Source: CAD feature listing. Evaluate the final solid. Frame: model axes, mm. A direction names the side the tool comes from. Coordinates: 2 decimals unless noted, no trailing zeros. Loops run counter-clockwise (first coordinate to the right, second up) from the corner with the lowest first, then second, coordinate; pieces in that order, holes last.
Item 1: Section query A-A, the plane x = 9. Return the cut outline in (y, z), then the cut area to 3 significant figures.
Item 2: Line query: probe 1 along Y at (x, z) = (9, 5.3); probe 2 along Z at (x, y) = (2.5, 135.5); probe 3 along Y at (x, z) = (9, 0.85). Output: solid intervals per line, ascending.
Item 3: Section query C-C, the plane y = 10. Return the cut outline in (x, z), then the cut area to 3 significant figures.
Item 4: Section query D-D, the plane x = 22.5. Return the cut outline in (y, z).
Item 5: Pull-direction query (X, two-part tool) for faces 6 (the cylindrical face through (8.874, 18.202, 1.812)), 7 (the cylindrical face through (7.568, 140.906, 4.535)), 8 (the flat face through (9, 125, 2)), 9 (the cylindrical face through (16, 1, 3)); classes: +X half, -X half, draft (parallel to the pull), parting line (faces both ways), or undercut.
Item 6: Pin query (flat end, axial travel): pin 1 Ø3.5 at (y, z) = (16, 3.5) entering from +X; pin 2 Ø4 at (y, z) = (102, 4.5) entering from -X; pin 3 Ø0.8 at (x, y) = (14.5, 135.5) entering from +Z. Return the tip coordinate at first contact, or that it passes through.
Item 7: Section query B-B, the plane y = 130. Return the cut outline in (x, z), then the cut area to 3 significant figures.
Item 8: Reachability of faces 1 (the flat face through (9, 8, 2.5)), 2 (the flat face through (18, 14, 3)), 3 (the flat face through (0, 14, 3)), 4 (the flat face through (9, 86, 7)), 5 (the flat face through (9, 8, 4.5)) from +Z, -Z, +X, -X, +Y, -Y: full face, straight path, thin tool, end or side. Return the list, or none.
```python
from build123d import *

# Parameters (mm, degrees)
ESQUISSE1_R             = 4.5
ESQUISSE1_W             = 18
ESQUISSE1_H             = 20
BOSS_EXTRU_1_DEPTH      = 7
ESQUISSE2_R             = 11
ENL_V_MAT_EXTRU_1_DEPTH = 5
ESQUISSE3_R             = 0.5
BOSS_EXTRU_2_DEPTH      = 3
ESQUISSE4_W             = 18
ESQUISSE4_H             = 20
ENL_V_MAT_EXTRU_2_DEPTH = 2.5
ESQUISSE5_W             = 18
ESQUISSE5_H             = 20
ENL_V_MAT_EXTRU_3_DEPTH = 2.5
CONG_1_R                = 5
CONG_2_R                = 15


with BuildPart() as part:
    # Esquisse1 → Boss.-Extru.1 (new body)
    # profile 1 of 2: a face of its own
    with BuildSketch(Plane.XY):
        Polygon((18, 20), (28, 150), (18, 150), (0, 150), (-10, 150), (0, 20), align=None)
        with Locations((9, 130)):
            Circle(ESQUISSE1_R, mode=Mode.SUBTRACT)
    # profile 2 of 2: a face of its own
    with BuildSketch(Plane.XY):
        with Locations((9, 10)):
            Rectangle(ESQUISSE1_W, ESQUISSE1_H)
    extrude(amount=BOSS_EXTRU_1_DEPTH)

    # Esquisse2 → Enlèv. mat.-Extru.1 (cut)
    with BuildSketch(Plane.XY.offset(7)):
        with Locations((9, 130)):
            Circle(ESQUISSE2_R)
    extrude(amount=-ENL_V_MAT_EXTRU_1_DEPTH, mode=Mode.SUBTRACT)

    # Esquisse3 → Boss.-Extru.2 (add)
    with BuildSketch(Plane.XY.offset(2)):
        with Locations((3.5, 135.5)):
            Circle(ESQUISSE3_R)
        with Locations((5.974873734, 137.974873734)):
            Circle(ESQUISSE3_R)
        with Locations((1.025126266, 133.025126266)):
            Circle(ESQUISSE3_R)
        with Locations((1.025126266, 126.974873734)):
            Circle(ESQUISSE3_R)
        with Locations((3.5, 124.5)):
            Circle(ESQUISSE3_R)
        with Locations((5.974873734, 122.025126266)):
            Circle(ESQUISSE3_R)
        with Locations((12.025126266, 122.025126266)):
            Circle(ESQUISSE3_R)
        with Locations((14.5, 124.5)):
            Circle(ESQUISSE3_R)
        with Locations((16.974873734, 126.974873734)):
            Circle(ESQUISSE3_R)
        with Locations((16.974873734, 133.025126266)):
            Circle(ESQUISSE3_R)
        with Locations((14.5, 135.5)):
            Circle(ESQUISSE3_R)
        with Locations((12.025126266, 137.974873734)):
            Circle(ESQUISSE3_R)
    extrude(amount=BOSS_EXTRU_2_DEPTH)

    # Esquisse4 → Enlèv. mat.-Extru.2 (cut)
    with BuildSketch(Plane.XY.offset(7)):
        with Locations((9, 10)):
            Rectangle(ESQUISSE4_W, ESQUISSE4_H)
    extrude(amount=-ENL_V_MAT_EXTRU_2_DEPTH, mode=Mode.SUBTRACT)

    # Esquisse5 → Enlèv. mat.-Extru.3 (cut)
    with BuildSketch(Plane(origin=(0, 0, 0), x_dir=(-1, 0, 0), z_dir=(0, 0, -1))):
        with Locations((-9, 10)):
            Rectangle(ESQUISSE5_W, ESQUISSE5_H)
    extrude(amount=-ENL_V_MAT_EXTRU_3_DEPTH, mode=Mode.SUBTRACT)

    # Congé1
    # the kernel refuses this fillet: 5 mm, written as the material it adds along each edge
    with BuildSketch(Plane(origin=(0, 20, 2.5), x_dir=(0, 0, -1), z_dir=(1, 0, 0)), Plane(origin=(18, 20, 4.5), x_dir=(0, 0, 1), z_dir=(-1, 0, 0))) as cong_1_piece_1:
        with BuildLine():
            CenterArc((5, -4.330127019), CONG_1_R, 120, 60)
            Line((0, -4.330127019), (0, 0))
            Line((0, 0), (2.5, 0))
        make_face()
    extrude(amount=18)
    # the kernel refuses this fillet: 5 mm, written as the material it takes off along each edge
    with BuildSketch(Plane(origin=(18, 0, -10), x_dir=(-1, 0, 0), z_dir=(0, 0, 1)), Plane(origin=(0, 0, -10), x_dir=(0, 1, 0), z_dir=(0, 0, 1))) as cong_1_2_piece_1:
        with BuildLine():
            CenterArc((CONG_1_R, -CONG_1_R), CONG_1_R, 90, 90)
            Line((0, -CONG_1_R), (0, 0))
            Line((0, 0), (CONG_1_R, 0))
        make_face()
    extrude(amount=27, mode=Mode.SUBTRACT)

    # Congé2
    cong_2_edges = [part.edges().sort_by_distance(p)[0] for p in [
        (-10, 150, 3.5),
        (28, 150, 3.5),
    ]]
    fillet(cong_2_edges, radius=CONG_2_R)


solid = part.part
```
Verdict:
1. outline: (0, 2.5) - (15.67, 2.5) arc R5 cw to (20, 0) - (125.5, 0) - (125.5, 2) - (119, 2) - (119, 7) - (20, 7) arc R5 cw to (15.67, 4.5) - (0, 4.5) - close; (134.5, 0) - (150, 0) - (150, 7) - (141, 7) - (141, 2) - (134.5, 2) - close
1. area: 828 mm2
2. probe 1: y = 18.38 to 119, 141 to 150
2. probe 2: z = 0 to 2
2. probe 3: y = 19.38 to 125.5, 134.5 to 150
3. outline: (0, 2.5) - (18, 2.5) - (18, 4.5) - (0, 4.5) - close
3. area: 36.0 mm2
4. outline: (78.5, 0) - (145.51, 0) - (145.51, 7) - (78.5, 7) - close
5. face 6: draft
5. face 7: undercut
5. face 8: undercut
5. face 9: +X half
6. pin 1: stops at x = 18
6. pin 2: stops at x = -6.46
6. pin 3: stops at z = 5
7. outline: (-8.46, 0) - (4.5, 0) - (4.5, 2) - (-2, 2) - (-2, 7) - (-8.46, 7) - close; (13.5, 0) - (26.46, 0) - (26.46, 7) - (20, 7) - (20, 2) - (13.5, 2) - close
7. area: 116 mm2
8. face 1: -Z, +X, -X, -Y
8. face 2: +Z, -Z, +X, -Y
8. face 3: +Z, -Z, -X, -Y
8. face 4: +Z, +X, -X, +Y, -Y
8. face 5: +Z, +X, -X, -Y
